Autodesk Inventor part; units mm, degrees
ref_plane "YZ Plane" through (0, 0, 0) normal (1, 0, 0) x (0, 1, 0)
ref_plane "XZ Plane" through (0, 0, 0) normal (0, 1, 0) x (-1, 0, 0)
ref_plane "XY Plane" through (0, 0, 0) normal (0, 0, 1) x (1, 0, 0)
sketch "Sketch6" plane through (0, 0, 0) normal (0, 0, 1) x (1, 0, 0)
  line L0 (90, 0) -> (90, 25)
  line L1 (90, 25) -> (129, 25)
  line L2 (129, 25) -> (129, 3)
  line L3 (129, 3) -> (132.5, 3)
  line L4 (132.5, 3) -> (132.5, 0)
  line L5 (132.5, 0) -> (90, 0)
  line L6 (0, 0) -> (0, 25)
  point P0 (0, 0)
  dimension "d27" = 180
  dimension "d28" = 258
  dimension "d29" = 265
  dimension "d30" = 3
  dimension "d31" = 25
revolve "Revolution1" add sketch "Sketch6" angle 360 about axis through (0, 0, 0) along (0, 1, 0)
sketch "Sketch7" plane through (0, 25, 0) normal (0, 1, 0) x (1, 0, 0)
  circle A0 centre (0, 0) radius 110
  point P0 (0, 110)
  dimension "d33" = 220
hole "Hole2" at (0, 25, -110) direction (0, -1, 0) diameter 11 end through all counterbore diameter 25 counterbore depth 10
pattern_circular "Circular Pattern3" count 8 over 360 about axis through (0, -10, 0) along (0, 1, 0) of "Hole2"
equation "\"d39\" = Thickness"
properties part number "DMF 01 31 Барабан Опорное кольцо НОС v2.1"
Read the model definition and answer for the solid it produces. Units are mm, in the model's axes. A direction names the side the tool comes from. Round coordinates to 2 decimals unless told otherwise and drop trailing zeros. Write each loop counter-clockwise with the first axis right and the second up, starting at its lowest first coordinate (ties: lowest second). Pieces come first, ordered by that corner, then holes. Notation, with made-up numbers: M -34,44 L 6,44 A29 cw 6,82 Z; hole C -14.75,6 d4. An arc over 180 degrees is marked long. Use a Markdown table: item, result.
1) The part is cut by section A-A (x = 0). Write down the section's boundary in (y, z), plus the area to 3 significant figures.
Answers follow:
| item | result |
|---|---|
| outline | M 0,-132.5 L 3,-132.5 L 3,-129 L 25,-129 L 25,-122.5 L 15,-122.5 L 15,-115.5 L 0,-115.5 Z; M 0,-104.5 L 15,-104.5 L 15,-97.5 L 25,-97.5 L 25,-90 L 0,-90 Z; M 0,90 L 25,90 L 25,97.5 L 15,97.5 L 15,104.5 L 0,104.5 Z; M 0,115.5 L 15,115.5 L 15,122.5 L 25,122.5 L 25,129 L 3,129 L 3,132.5 L 0,132.5 Z |
| area | 1,140 mm2 |
2) A tool of negligible diameter and unlimited length cuts with its end or side. For faces 4 (the cylindrical face through (41.53, 12.675, 79.845)), 5 (the cylindrical face through (3.755, 19.93, 98.077)), from which of +Z, -Z, +X, -X, +Y, -Y can it reach the whole face along a straight path? Write none if from no direction.
Answers follow:
| item | result |
|---|---|
| face 4 | +Y, -Y |
| face 5 | +Y |
3) Straight lines are drawn through the part: line 1 along X through (y, z) = (14, -0.5); line 2 along X through (y, z) = (19, 72); line 3 along X through (y, z) = (11.25, -110). For each, find the intervals that lie inside material, in ascending order. Write a range as [from, to].
Answers follow:
| item | result |
|---|---|
| line 1 | x = [-129, -115.48], [-104.52, -90], [90, 104.52], [115.48, 129] |
| line 2 | x = [-107.04, -88.86], [-66.7, -54], [54, 66.7], [88.86, 107.04] |
| line 3 | x = [-67.39, -5.5], [5.5, 67.39] |
4) The part is cut by section C-C (x = -108). Write down the section's boundary in (y, z), plus the area to 3 significant figures.
Answers follow:
| item | result |
|---|---|
| outline | M 0,-76.76 L 3,-76.76 L 3,-70.55 L 25,-70.55 L 25,-12.34 L 15,-12.34 L 15,-5.12 L 0,-5.12 Z; M 0,5.12 L 15,5.12 L 15,12.34 L 25,12.34 L 25,70.55 L 3,70.55 L 3,76.76 L 0,76.76 Z |
| area | 3,160 mm2 |
5) The part is cut by section D-D (z = 29). Write down the section's boundary in (x, y), plus the area to 3 significant figures.
Answers follow:
| item | result |
|---|---|
| outline | M -129.29,0 L -85.2,0 L -85.2,25 L -125.7,25 L -125.7,3 L -129.29,3 Z; M 85.2,0 L 129.29,0 L 129.29,3 L 125.7,3 L 125.7,25 L 85.2,25 Z |
| area | 2,050 mm2 |
6) Flat-ended cylindrical pins translate along their axes: pin 1 (20 mm diameter, centred on x = -78.5, z = -78, fed in from +Y); pin 2 (12 mm diameter, centred on y = 17.5, z = 59, fed in from +X); pin 3 (10 mm diameter, centred on x = -48.5, y = 22.5, fed in from +Z). Find the tip coordinate at first contact, or state that the pin passes through.
Answers follow:
| item | result |
|---|---|
| pin 1 | stops at y = 15 |
| pin 2 | stops at x = 117.61 |
| pin 3 | stops at z = 121.44 |
7) For a pull along Z with two mould halves and no side action, classify faces 1 (the cylindrical face through (123.043, 13.846, 38.748)), 2 (the flat face through (29, 3, 127)), 3 (the cylindrical face through (-115.495, 7.395, 0.242)) as pulls with the +Z half, pulls with the -Z half, needs draft (parallel to the pull), parting line crosses it, or undercut.
Answers follow:
| item | result |
|---|---|
| face 1 | parting line crosses it |
| face 2 | needs draft |
| face 3 | undercut |
8) The part is cut by section B-B (z = 110). Write down the section's boundary in (x, y), plus the area to 3 significant figures.
Answers follow:
| item | result |
|---|---|
| outline | M -73.87,0 L -5.5,0 L -5.5,15 L -12.5,15 L -12.5,25 L -67.39,25 L -67.39,3 L -73.87,3 Z; M 5.5,0 L 73.87,0 L 73.87,3 L 67.39,3 L 67.39,25 L 12.5,25 L 12.5,15 L 5.5,15 Z |
| area | 2,990 mm2 |
